from build123d import *

# Parameters (mm, degrees)
BOSS_EXTRUDE1_DEPTH = 2
SKETCH2_W           = 0.5
SKETCH2_H           = 3.8
SKETCH3_W           = 0.5
SKETCH3_H           = 3.8
SKETCH4_W           = 0.5
SKETCH4_H           = 3.8
FILLET1_R           = 3
FILLET2_R           = 20


with BuildPart() as part:
    # Sketch1 → Boss-Extrude1 (new body)
    with BuildSketch(Plane.XY.offset(2)):
        with BuildLine():
            Line((7.771354167, 22.540832259), (-27.228645833, 22.540832259))
            Line((-27.228645833, 22.540832259), (-27.228645833, -27.813067392))
            add(Edge.make_bspline(
                [(-27.228645833, -27.813067392), (-26.427873486, -29.29582054), (-25.627101139, -30.778573688), (-24.826328792, -32.261326836), (-19.837606386, -41.498713565), (-9.897506481, -50.952288279), (1.392273584, -41.560087902), (5.904599103, -31.862127656), (6.526850791, -30.524774642), (7.149102479, -29.187421629), (7.771354167, -27.850068615)],
                knots=[0, 0, 0, 0, 0.06863763, 0.06863763, 0.06863763, 0.496242407, 0.937653653, 0.937653653, 0.937653653, 0.998524459, 0.998524459, 0.998524459, 0.998524459], degree=3))
            Line((7.771354167, -27.850068615), (7.771354167, 22.540832259))
        make_face()
    extrude(amount=-BOSS_EXTRUDE1_DEPTH)

    # Sketch2 → Revolve1 (revolve)
    with BuildSketch(Plane.XZ.offset(22.757561557), mode=Mode.PRIVATE) as revolve1_sk:
        with Locations((7.021354167, 3.9)):
            Rectangle(SKETCH2_W, SKETCH2_H)
    revolve(revolve1_sk.sketch.rotate(Axis((6.771354167, -22.757561557, 5.8), (0, 0, -1)), 180), axis=Axis((6.771354167, -22.757561557, 5.8), (0, 0, -1)))

    # Sketch3 → Revolve2 (revolve)
    with BuildSketch(Plane.XZ.offset(22.757561557), mode=Mode.PRIVATE) as revolve2_sk:
        with Locations((-25.978645833, 3.9)):
            Rectangle(SKETCH3_W, SKETCH3_H)
    revolve(revolve2_sk.sketch.rotate(Axis((-26.228645833, -22.757561557, 5.8), (0, 0, -1)), 180), axis=Axis((-26.228645833, -22.757561557, 5.8), (0, 0, -1)))

    # Sketch4 → Revolve3 (revolve)
    with BuildSketch(Plane.XZ.offset(-21.540832259), mode=Mode.PRIVATE) as revolve3_sk:
        with Locations((-9.478645833, 3.9)):
            Rectangle(SKETCH4_W, SKETCH4_H)
    revolve(revolve3_sk.sketch.rotate(Axis((-9.728645833, 21.540832259, 5.8), (0, 0, -1)), 180), axis=Axis((-9.728645833, 21.540832259, 5.8), (0, 0, -1)))

    # Fillet1
    fillet1_edges = [part.edges().sort_by_distance(p)[0] for p in [
        (-27.228645833, 22.540832259, 1),
        (7.771354167, 22.540832259, 1),
    ]]
    fillet(fillet1_edges, radius=FILLET1_R)

    # Fillet2
    fillet2_edges = [part.edges().sort_by_distance(p)[0] for p in [
        (7.771354167, -27.850068615, 1),
        (-27.228645833, -27.813067392, 1),
    ]]
    fillet(fillet2_edges, radius=FILLET2_R)


solid = part.part
Verification items for the finished model (mm, model axes). Coordinates: 2 decimals unless noted, no trailing zeros. Order: outer loops, then holes, each group sorted by start corner. A loop starts at its lowest first (then second) coordinate and runs counter-clockwise, first axis right, second up. Notation, with made-up numbers: M 56.5,-25.75 L 67.5,-25.75 A12 cw 67.5,-5.75 Z; hole C 70,87 d11. An arc over 180 degrees is marked long. Return JSON: item names as keys, results as strings.
1) Cross-section at B-B, the plane y = 1. Record the boundary of the cut face in (x, z), and give its area (3 significant figures).
Answer list:
{"outline": "M -27.23,0 L 7.77,0 L 7.77,2 L -27.23,2 Z", "area": "70.0 mm2"}
2) Gauge pin test, flat end, axial feed: pin 1 (10.5 mm diameter, centred on x = -2, y = -0.5, fed in from +Z). Record the tip position at first contact, or that the pin passes through.
Answer list:
{"pin 1": "z = 2"}
3) Cross-section at A-A, the plane z = 4. Record the boundary of the cut face in (x, y).
Answer list:
{"outline": "C -26.23,-22.76 d1; C -9.73,21.54 d1; C 6.77,-22.76 d1"}
4) Thickness scan on L1, parallel to Z at x = -18, y = -18; L2, parallel to Y at x = -8, z = 0.75; L3, parallel to X at y = -41.5, z = 0.45. Record the ranges inside material, lowest first. Write a range as [from, to].
Answer list:
{"L1": "[0, 2]", "L2": "[-46.1, 22.54]", "L3": "[-18.54, -0.33]"}
